Autodesk Inventor part; units mm, degrees
ref_plane "Work Plane1" through (-5.335, -17.8017, 25) normal (0, -1, 0) x (1, 0, 0)
ref_plane "YZ Plane" through (0, 0, 0) normal (1, 0, 0) x (0, 1, 0)
ref_plane "XZ Plane" through (0, 0, 0) normal (0, 1, 0) x (-1, 0, 0)
sketch "Sketch2" plane through (0, 0, 0) normal (0, 0, 1) x (1, 0, 0)
  line L0 (-5.335, -2.8017) -> (69.665, -2.8017)
  line L1 (69.665, -2.8017) -> (69.665, -32.8017)
  line L2 (69.665, -32.8017) -> (-5.335, -32.8017)
  line L3 (-5.335, -32.8017) -> (-5.335, -2.8017)
  dimension "d0" = 30
  dimension "d1" = 75
extrude "Extrusion1" add sketch "Sketch2" along normal blind 25
sketch "Sketch3" plane through (-5.335, -32.8017, 0) normal (-1, 0, 0) x (0, 0, 1)
  line L0 (25, 0) -> (25, 30)
  line L1 (0, 30) -> (25, 30)
  line L2 (0, 0) -> (0, 30)
  line L3 (0, 0) -> (25, 0)
  line L4 (25, 30) -> (80, 30)
  arc A0 (80, 0) -> (80, 30) centre (80, 15) ccw
  line L5 (80, 0) -> (25, 0)
  dimension "d15" = 80
extrude "Extrusion2" add sketch "Sketch3" along normal blind 25
sketch "Sketch5" plane through (69.665, -32.8017, 0) normal (1, 0, 0) x (0, 0, -1)
  line L0 (0, 0) -> (-25, 0)
  line L1 (0, 30) -> (0, 0)
  line L2 (-6, 0) -> (-11, 0)
  line L3 (-11, 0) -> (-11, 6)
  line L4 (-11, 6) -> (-6, 6)
  line L5 (-6, 6) -> (-6, 0)
  dimension "d16" = 5
  dimension "d17" = 6
  dimension "d18" = 6
extrude "Extrusion4" cut sketch "Sketch5" against normal through all
ref_plane "Work Plane1" through (-5.335, -17.8017, 25) normal (0, -1, 0) x (1, 0, 0)
mirror "Mirror1" about plane through (-5.335, -17.8017, 25) normal (0, -1, 0) of "Extrusion4"
fillet "Fillet1" radius 15 1 edges at (-5.335, -17.8017, 25)
sketch "Sketch4" plane through (0, 0, 25) normal (0, 0, 1) x (1, 0, 0)
  line L0 (19.665, -13.3017) -> (59.665, -13.3017)
  arc A0 (59.665, -22.3017) -> (59.665, -13.3017) centre (59.665, -17.8017) ccw
  line L1 (59.665, -22.3017) -> (19.665, -22.3017)
  arc A1 (19.665, -13.3017) -> (19.665, -22.3017) centre (19.665, -17.8017) ccw
  line L2 (-30.335, -32.8017) -> (-30.335, -2.8017)
  line L3 (69.665, -32.8017) -> (9.665, -32.8017)
  line L4 (69.665, -2.8017) -> (69.665, -32.8017)
  dimension "d10" = 4.5
  dimension "d12" = 50
  dimension "d21" = 15
  dimension "d22" = 10
extrude "Extrusion3" cut sketch "Sketch4" against normal through all
chamfer "Chamfer2" distance 5 angle 45 4 edges at (69.665, -2.8017, 18) (69.665, -32.8017, 18) (69.665, -2.8017, 3) (69.665, -32.8017, 3)
sketch "Sketch9" plane through (-30.335, -32.8017, 0) normal (-1, 0, 0) x (0, 0, 1)
  line L0 (0, 0) -> (0, 30)
  line L1 (80, 0) -> (11, 0)
  point P0 (75, 15)
  point P1 (40, 15)
  dimension "d50" = 15
  dimension "d51" = 75
  dimension "d52" = 40
hole "Hole4" at (-30.335, -17.8017, 75) at (-30.335, -17.8017, 40) direction (1, 0, 0) diameter 6.647 end through all
equation "\"d21\" = 0.5 * d0"
properties part number "100006"
The listing builds one solid part. Answer for the finished solid, in the listing's coordinates (mm). A direction names the side the tool comes from. Round coordinates to 2 decimals unless told otherwise and drop trailing zeros. Write each loop counter-clockwise with the first axis right and the second up, starting at its lowest first coordinate (ties: lowest second). Pieces come first, ordered by that corner, then holes. Notation, with made-up numbers: (5, -27) -> (20, -27) arc R24 ccw to (20, -4) -> close; hole circle Ø11 at (63, 84.5). An arc over 180 degrees is marked (long way). Write item = value, one per line.
1) For a pull along Y with two mould halves and no side action, classify faces 5 (the flat face through (20, -8.802, 8)), 6 (the cylindrical face through (64.164, -17.901, 12.675)), 7 (the flat face through (18, -32.802, 3)) as released by +Y, released by -Y, zero draft, split by the parting line, or undercut.
Check values:
face_5 = released by +Y
face_6 = undercut
face_7 = released by -Y
2) Section B-B on z = 75 is taken. Write down the section's boundary in (x, y) (3 decimals).
Check values:
outline = (-30.335, -32.802) -> (-5.335, -32.802) -> (-5.335, -21.125) -> (-30.335, -21.125) -> close; (-30.335, -14.478) -> (-5.335, -14.478) -> (-5.335, -2.802) -> (-30.335, -2.802) -> close
3) Given pin 1 (5 mm diameter, centred on x = -0.5, y = -29, fed in from +Z); pin 2 (5 mm diameter, centred on x = 11.5, y = -5.5, fed in from +Z); pin 3 (2.5 mm diameter, centred on x = 8, z = 9, fed in from -Y), each flat-ended and moving along its own axis, determine where each tip first touches the part or whether it passes through.
Check values:
pin_1 = 31.96
pin_2 = 25.01
pin_3 = -26.8
4) Section D-D on z = 20 is taken. Write down the section's boundary in (x, y) (3 decimals).
Check values:
outline = (-30.335, -32.802) -> (64.665, -32.802) -> (69.665, -27.802) -> (69.665, -7.802) -> (64.665, -2.802) -> (-30.335, -2.802) -> close; hole (19.665, -22.302) -> (59.665, -22.302) arc R4.5 ccw to (59.665, -13.302) -> (19.665, -13.302) arc R4.5 ccw to start
5) Section A-A on x = 40.5 is taken. Write down the section's boundary in (y, z).
Check values:
outline = (-32.8, 0) -> (-22.3, 0) -> (-22.3, 25) -> (-32.8, 25) -> (-32.8, 11) -> (-26.8, 11) -> (-26.8, 6) -> (-32.8, 6) -> close; (-13.3, 0) -> (-2.8, 0) -> (-2.8, 6) -> (-8.8, 6) -> (-8.8, 11) -> (-2.8, 11) -> (-2.8, 25) -> (-13.3, 25) -> close
6) Straight lines are drawn through the part: line 1 along Z through (x, y) = (46, -5); line 2 along Y through (x, z) = (43.5, 8); line 3 along Y through (x, z) = (49.5, 16). For each, find the intervals that lie inside material, in ascending order. Write a range as [from, to].
Check values:
line_1 = [0, 6], [11, 25]
line_2 = [-26.8, -22.3], [-13.3, -8.8]
line_3 = [-32.8, -22.3], [-13.3, -2.8]
7) Section C-C on y = -5.5 is taken. Write down the section's boundary in (x, z) (3 decimals), plus the area to 3 significant figures.
Check values:
outline = (-30.335, 0) -> (67.363, 0) -> (67.363, 6) -> (-30.335, 6) -> close; (-30.335, 11) -> (67.363, 11) -> (67.363, 25) -> (9.665, 25) arc R15 cw to (-5.335, 40) -> (-5.335, 88.583) -> (-30.335, 88.583) -> close
area = 3,590 mm²
8) Which of the six approach directions +Z, -Z, +X, -X, +Y, -Y give full straight-line access (tool end or side, diameter ignored) to faces 1 (the flat face through (-5.335, -18, 67)), 2 (the flat face through (20, -6, 11)), 3 (the flat face through (40, -22.302, 13)), 4 (the flat face through (20, -30, 6))?
Check values:
face_1 = +Z, +X, +Y, -Y
face_2 = +X, -X, +Y
face_3 = +Z, -Z
face_4 = +X, -X, -Y
